Work out the finished part from the listing and answer in its coordinate system (mm). A direction names the side the tool comes from. Give positions to 0.01 mm unless a question says otherwise; leave off trailing zeros. Loops run counter-clockwise (first coordinate to the right, second up) from the corner with the lowest first, then second, coordinate; pieces in that order, holes last. Notation, with made-up numbers: (-10.5, 47) - (32.5, 47) arc R25 cw to (32.5, 70) - close; hole circle Ø9 at (39.25, 35.5). An arc over 180 degrees is marked (long way). One line per item, written item: value.
from build123d import *

# Parameters (mm, degrees)
BOSS_EXTRUDE1_DEPTH = 2636.78
SKETCH2_W           = 193.333333334
SKETCH2_H           = 300
BOSS_EXTRUDE2_DEPTH = 15
SKETCH3_W           = 193.333
SKETCH3_H           = 300
BOSS_EXTRUDE4_DEPTH = 15


with BuildPart() as part:
    # Sketch1 → Boss-Extrude1 (new body)
    with BuildSketch(Plane.XY):
        Polygon((-13.333333333, -4.45387532), (-13.333333333, 145.54612468), (-96.666333333, 145.54612468), (-96.666333333, 162.212791347), (-13.333333333, 162.212791347), (0, 162.212791347), (96.666666667, 162.212791347), (96.666666667, 145.54612468), (13.333333333, 145.54612468), (13.333333333, -154.45387532), (96.666666667, -154.45387532), (96.666666667, -171.120541986), (-96.666666667, -171.120541986), (-96.666666667, -154.45387532), (-13.333333333, -154.45387532), align=None)
    extrude(amount=BOSS_EXTRUDE1_DEPTH)

    # Sketch2 → Boss-Extrude2 (add)
    with BuildSketch(Plane(origin=(0, 0, 0), x_dir=(-1, 0, 0), z_dir=(0, 0, -1))):
        with Locations((0, -4.45387532)):
            Rectangle(SKETCH2_W, SKETCH2_H)
    extrude(amount=-BOSS_EXTRUDE2_DEPTH)

    # Sketch3 → Boss-Extrude4 (add)
    with BuildSketch(Plane.XY.offset(2636.78)):
        with Locations((0.000166667, -4.45387532)):
            Rectangle(SKETCH3_W, SKETCH3_H)
    extrude(amount=-BOSS_EXTRUDE4_DEPTH)


solid = part.part
1. Section A-A (z = 1884) is taken. Write down the section's boundary in (x, y).
Output:
outline: (-96.67, -171.12) - (96.67, -171.12) - (96.67, -154.45) - (13.33, -154.45) - (13.33, 145.55) - (96.67, 145.55) - (96.67, 162.21) - (-96.67, 162.21) - (-96.67, 145.55) - (-13.33, 145.55) - (-13.33, -154.45) - (-96.67, -154.45) - close
2. For faces 1 (the flat face through (54, -2, 2621.78)), 2 (the flat face through (1, 162.213, 1300)), 3 (the flat face through (-13.333, -2, 1300)), determine the directions among +Z, -Z, +X, -X, +Y, -Y from which every point of the face is accessible in a straight line to the end or side of a thin tool.
Output:
face 1: +X
face 2: +Z, -Z, +X, -X, +Y
face 3: -X
3. Section B-B (x = 58.5) is taken. Write down the section's boundary in (y, z).
Output:
outline: (-171.12, 0) - (162.21, 0) - (162.21, 2636.78) - (-171.12, 2636.78) - close; hole (-154.45, 15) - (145.55, 15) - (145.55, 2621.78) - (-154.45, 2621.78) - close
4. The mould has two halves that part along Y. Classify faces 4 (the flat face through (-96.666, 156, 1325)), 5 (the flat face through (-56, -2, 2621.78)), 6 (the flat face through (1, -171.121, 1300)), 7 (the flat face through (-54, 145.546, 1300)): released by +Y, released by -Y, zero draft, split by the parting line, or undercut.
Output:
face 4: zero draft
face 5: undercut
face 6: released by -Y
face 7: undercut
5. Section C-C (y = 115.5) is taken. Write down the section's boundary in (x, z), and give its area (3 significant figures).
Output:
outline: (-96.67, 0) - (96.67, 0) - (96.67, 15) - (13.33, 15) - (13.33, 2621.78) - (96.67, 2621.78) - (96.67, 2636.78) - (-96.67, 2636.78) - (-96.67, 2621.78) - (-13.33, 2621.78) - (-13.33, 15) - (-96.67, 15) - close
area: 75,300 mm²
6. Find the intervals of material crossed by line 1 along Y through (x, z) = (24, 1156); line 2 along Z through (x, y) = (68, -5.5); line 3 along X through (y, z) = (-3, 2317), in increasing order.
Output:
line 1: y = -171.12 to -154.45, 145.55 to 162.21
line 2: z = 0 to 15, 2621.78 to 2636.78
line 3: x = -13.33 to 13.33
